Design review of the part built by this model. Coordinates are the model's own, in mm. Face numbers are marked on the shaded views. A direction names the side the tool comes from. Coordinates: 2 decimals unless noted, no trailing zeros. Loops run counter-clockwise (first coordinate to the right, second up) from the corner with the lowest first, then second, coordinate; pieces in that order, holes last. Notation, with made-up numbers: (77.5, 62) -> (105.5, 62) arc R21 cw to (105.5, 67) -> close; hole circle Ø2 at (-37.5, 58). An arc over 180 degrees is marked (long way). One line per item, written item: value. Start each with the question number.
1. Machinability: for the marked faces 1, 2 and 3, which of the approach directions +Z, -Z, +X, -X, +Y, -Y give a long, thin tool a straight path to every point of the face, cutting with its end or side? Answer none if there is none.
2. Draft analysis for pull direction X (two halves, no side actions). For the marked faces 4, 5, 6 and 7, state which applies: pulls with the +X half, pulls with the -X half, needs draft (parallel to the pull), parting line crosses it, or undercut.
3. For probe 1 along Y at (x, z) = (5, -9.25); probe 2 along Y at (x, z) = (-11, -4.25); probe 3 along Z at (x, y) = (0, -6.9), list the stretches that pass through material, from the lowest coordinate up.
4. Add section A-A on z = 0. Give the number of separate pieces and of enclosed holes in the cut face, plus the area to 3 significant figures.
5. Add section B-B on x = -6. Write out the cut boundary in (y, z).
6. Insertion check: pin 1 (2 mm diameter, centred on y = -54.5, z = -9, fed in from +X); pin 2 (0.8 mm diameter, centred on x = -17, z = 0, fed in from -Y); pin 3 (1.2 mm diameter, centred on x = -11.5, y = -45, fed in from +Z). Each pin has a flat end and moves straight along its axis. Give the tip position at first contact, or say it passes through.
7. Add section C-C on y = -25. Write out the cut boundary in (x, z), plus the area to 3 significant figures.
8. Add section D-D on z = -13. Write out the cut boundary in (x, y).
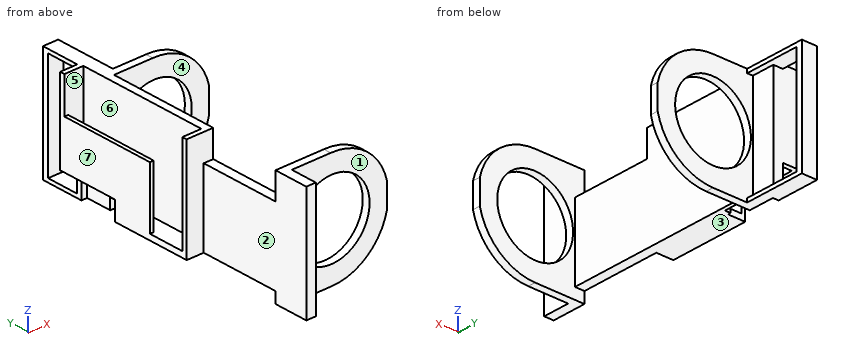
Autodesk Inventor part; units mm, degrees
ref_plane "YZ Plane" through (0, 0, 0) normal (1, 0, 0) x (0, 1, 0)
ref_plane "XZ Plane" through (0, 0, 0) normal (0, 1, 0) x (-1, 0, 0)
ref_plane "XY Plane" through (0, 0, 0) normal (0, 0, 1) x (1, 0, 0)
sketch "Sketch1" plane through (0, 0, 0) normal (0, 1, 0) x (-1, 0, 0)
  line L0 (13, 14.9495) -> (0, 14.9495)
  line L1 (0, -14.9505) -> (13, -14.9505)
  line L2 (13, -14.9505) -> (13, 14.9495)
  arc A0 (-14.7414, -2.4918) -> (0, -14.9505) centre (0, 0) ccw
  arc A1 (0.2506, 14.9495) -> (-14.7414, -2.4918) centre (-0.0002, 0.001) ccw
  point P0 (13, -0.0005)
  dimension "d0" = 29.9
  dimension "d1" = 0
  dimension "d2" = 0
extrude "Extrusion1" add sketch "Sketch1" against normal blind 60
sketch "Sketch2" plane through (0, -60, 0) normal (0, -1, 0) x (1, 0, 0)
  circle A0 centre (0, 0) radius 10
  dimension "d5" = 20
extrude "Extrusion2" cut sketch "Sketch2" against normal through all
sketch "Sketch3" plane through (0, 0, 0) normal (0, 1, 0) x (1, 0, 0)
  line L0 (-13, -14.9495) -> (-13, 14.9505)
  line L1 (-0.2506, -14.9495) -> (-13, -14.9495)
  line L2 (-13, 14.9505) -> (-10.5, 14.9505)
  line L3 (-10.5, 14.9505) -> (-10.5, -14.9495)
  line L4 (-10.5, -14.9495) -> (-13, -14.9495)
  line L5 (-13, -14.9495) -> (-13, 14.9505)
  point P0 (0, 0)
  point P1 (0, -15)
  dimension "d8" = 2.5
extrude "Extrusion3" add sketch "Sketch3" against normal blind 67
sketch "Sketch4" plane through (-10.5, -67, 14.9495) normal (1, 0, 0) x (0, 0, -1)
  line L0 (-3.796, 59) -> (37.1499, 59)
  line L1 (37.1499, 59) -> (37.1499, 9)
  line L2 (37.1499, 9) -> (-3.796, 9)
  line L3 (-3.796, 9) -> (-3.796, 59)
  line L4 (29.9, 67) -> (0, 67)
  line L5 (0, 7) -> (29.9, 7)
  point P0 (14.9495, 67)
  dimension "d31" = 2
  dimension "d44" = 50
extrude "Extrusion4" cut sketch "Sketch4" along normal through all
sketch "Sketch5" plane through (0, 0, 0) normal (0, 1, 0) x (1, 0, 0)
  line L0 (-13, 14.9505) -> (-13, -14.9495)
  line L1 (-10.5, 14.9505) -> (0, 14.9505)
  line L2 (-13, -14.9495) -> (-9, -14.9495)
  line L3 (-9, -14.9495) -> (-9, 14.9505)
  line L4 (-9, 14.9505) -> (-13, 14.9505)
  line L5 (-13, 14.9505) -> (-13, -14.9495)
  point P0 (0, 0)
  dimension "d13" = 4
extrude "Extrusion5" add sketch "Sketch5" along normal blind 10
sketch "Sketch6" plane through (-9, 0, 4.3589) normal (1, 0, 0) x (0, 0, -1)
  line L0 (0, 0) -> (-10.5906, 0)
  line L1 (-9.5906, 0) -> (18.3094, 0)
  line L2 (18.3094, 0) -> (18.3094, 8.5)
  line L3 (18.3094, 8.5) -> (-9.5906, 8.5)
  line L4 (-9.5906, 8.5) -> (-9.5906, 0)
  line L5 (19.3094, 0) -> (19.3094, 10)
  line L6 (-10.5906, 0) -> (-10.5906, 10)
  line L7 (-10.5906, 10) -> (19.3094, 10)
  point P0 (4.3589, 0)
  point P1 (19.3094, 5)
  dimension "d35" = 1
  dimension "d36" = 1
  dimension "d37" = 1.5
extrude "Extrusion6" cut sketch "Sketch6" against normal through all
sketch "Sketch7" plane through (-13, -67, -14.9505) normal (-1, 0, 0) x (0, 0, 1)
  line L0 (29.9, 67) -> (2.9, 67)
  line L1 (2.9, 67) -> (2.9, 30)
  line L2 (2.9, 30) -> (29.9, 30)
  line L3 (29.9, 30) -> (29.9, 67)
  line L4 (28.9, 67) -> (1, 67)
  line L5 (29.9, 0) -> (29.9, 77)
  line L6 (0, 0) -> (0, 77)
  point P0 (14.9505, 67)
  dimension "d54" = 37
  dimension "d55" = 27
  dimension "d57" = 0
  dimension "d60" = 0
extrude "Extrusion7" add sketch "Sketch7" along normal blind 4.5
sketch "Sketch8" plane through (-17.5, -67, -14.9505) normal (-1, 0, 0) x (0, 0, 1)
  line L0 (4.4, 65.75) -> (29.9, 65.75)
  line L1 (29.9, 65.75) -> (29.9, 31.25)
  line L2 (29.9, 31.25) -> (4.4, 31.25)
  line L3 (4.4, 31.25) -> (4.4, 65.75)
  line L4 (29.9, 30) -> (29.9, 67)
  line L5 (2.9, 30) -> (29.9, 30)
  point P0 (14.9505, 67)
  dimension "d61" = 0
  dimension "d62" = 34.5
  dimension "d63" = 25.5
  dimension "d64" = 1.25
extrude "Extrusion8" cut sketch "Sketch8" against normal blind 5
sketch "Sketch10" plane through (-10.5, -67, 14.9495) normal (1, 0, 0) x (0, 0, -1)
  line L0 (1, 67) -> (28.9, 67)
  line L1 (28.9, 67) -> (28.9, 61)
  line L2 (28.9, 61) -> (1, 61)
  line L3 (1, 61) -> (1, 67)
  line L4 (30, 59) -> (0, 59)
  line L5 (29.9, 67) -> (29.9, 77)
  line L6 (0, 67) -> (0, 77)
  point P0 (14.9495, 67)
  point P1 (1, 64)
  dimension "d45" = 2
  dimension "d46" = 6
  dimension "d48" = 1
  dimension "d50" = 1
extrude "Extrusion10" cut sketch "Sketch10" along normal through all
sketch "Sketch11" plane through (-9, 0, -14.9505) normal (1, 0, 0) x (0, 0, -1)
  line L0 (0, -67) -> (0, 10)
  line L1 (-30, 0) -> (-30, -8)
  line L2 (0, 1.2785) -> (-30, 1.2785)
  line L3 (-30, 1.2785) -> (-30, -6)
  line L4 (-30, -6) -> (0, -6)
  line L5 (0, -6) -> (0, 1.2785)
  line L6 (0, -8) -> (-30, -8)
  point P0 (-14.9505, 0)
  point P1 (0, -6)
  dimension "d51" = 2
extrude "Extrusion11" cut sketch "Sketch11" along normal through all contours L4 L1 L3 L2 L0
sketch "Sketch12" plane through (-17.5, -67, -14.9505) normal (-1, 0, 0) x (0, 0, 1)
  line L0 (2.9, 30) -> (2.9, 67)
  line L1 (2.9, 67) -> (20.4, 67)
  line L2 (20.4, 67) -> (20.4, 40.75)
  line L3 (20.4, 40.75) -> (2.9, 40.75)
  line L4 (2.9, 40.75) -> (2.9, 67)
  line L5 (4.4, 31.25) -> (4.4, 65.75)
  line L6 (4.4, 65.75) -> (29.9, 65.75)
  point P0 (14.9505, 67)
  point P1 (2.9, 40.75)
  dimension "d67" = 16
  dimension "d68" = 25
extrude "Extrusion12" add sketch "Sketch12" against normal blind 1
sketch "Sketch13" plane through (-13, -35.75, 14.9495) normal (-1, 0, 0) x (0, 0, 1)
  line L0 (0, 0) -> (-25.5, 0)
  line L1 (0, 0) -> (-7, 0)
  line L2 (-7, 0) -> (-7, 13)
  line L3 (-7, 13) -> (0, 13)
  line L4 (0, 13) -> (0, 0)
  point P0 (-14.9495, 35.75)
  dimension "d76" = 7
  dimension "d77" = 13
extrude "Extrusion13" [suppressed]
sketch "Sketch14" plane through (-17.5, -67, -14.9505) normal (-1, 0, 0) x (0, 0, 1)
  line L0 (7.9, 67) -> (2.9, 67)
  line L1 (2.9, 67) -> (2.9, 51)
  line L2 (2.9, 51) -> (7.9, 51)
  line L3 (7.9, 51) -> (7.9, 67)
  line L4 (2.9, 67) -> (2.9, 30)
  line L5 (29.9, 67) -> (2.9, 67)
  point P0 (14.9505, 67)
  dimension "d73" = 16
  dimension "d74" = 0
  dimension "d75" = 5
  dimension "d113" = 0
extrude "Extrusion14" cut sketch "Sketch14" against normal up to surface (4.5 mm away)
sketch "Sketch15" plane through (-13, -67, -14.9505) normal (-1, 0, 0) x (0, 0, 1)
  line L0 (29.9, 9) -> (0, 9)
  line L1 (0, 59) -> (2.9, 59)
  line L2 (2.9, 59) -> (2.9, 9)
  line L3 (2.9, 9) -> (0, 9)
  line L4 (0, 9) -> (0, 59)
  line L5 (2.9, 51) -> (2.9, 30)
  line L6 (0, 0) -> (0, 77)
  point P0 (14.9505, 67)
  dimension "d90" = 0
  dimension "d91" = 0
extrude "Extrusion15" cut sketch "Sketch15" against normal through all
sketch "Sketch16" plane through (-13, -67, -14.9505) normal (-1, 0, 0) x (0, 0, 1)
  line L0 (29.9, 30) -> (2.9, 30)
  line L1 (29.9, 9) -> (22.9, 9)
  line L2 (22.9, 9) -> (22.9, 30)
  line L3 (22.9, 30) -> (29.9, 30)
  line L4 (29.9, 30) -> (29.9, 9)
  line L5 (29.9, 0) -> (29.9, 30)
  point P0 (14.9505, 67)
  dimension "d82" = 0
  dimension "d83" = 7
extrude "Extrusion16" cut sketch "Sketch16" against normal through all
sketch "Sketch18" plane through (-10.5, -6, 13.9495) normal (0, 1, 0) x (1, 0, 0)
  line L0 (26.137, 9.211) -> (25.1, 9.211)
  line L1 (25.1, 9.211) -> (25.1, 19.211)
  line L2 (25.1, 19.211) -> (26.137, 19.211)
  line L3 (26.137, 19.211) -> (26.137, 9.211)
  arc A0 (10.5, -1) -> (10.5, 29) centre (10.5, 14) ccw
  point P0 (10.5, 13.9495)
  point P1 (25.1, 14.211)
  point P2 (25.5, 14)
  point P3 (25.6185, 19.211)
  point P4 (25.6185, 9.211)
  dimension "d88" = 10
  dimension "d89" = 14.6
extrude "Extrusion17" cut sketch "Sketch18" against normal through all
sketch "Sketch19" plane through (-13, -8, -14.9505) normal (-1, 0, 0) x (0, 0, 1)
  line L0 (20.4, 6.75) -> (29.9, 6.75)
  line L1 (-1.6421, -7.2479) -> (7.9, -7.2479)
  line L2 (7.9, -7.2479) -> (7.9, 6.75)
  line L3 (7.9, 6.75) -> (-1.6421, 6.75)
  line L4 (-1.6421, 6.75) -> (-1.6421, -7.2479)
  point P0 (14.9505, 8)
  point P1 (2.9, 6.75)
  point P2 (2.9, 6.75)
extrude "Extrusion18" cut sketch "Sketch19" against normal blind 1.5
properties part number "Part4-2option"
Worked answers:
1. face 1: +Z, -Z, +X, -Y
1. face 2: +Z, -Z, -X, -Y
1. face 3: -Z, +X, -X
2. face 4: needs draft
2. face 5: undercut
2. face 6: undercut
2. face 7: pulls with the -X half
3. probe 1: y = -60 to -58, -8 to -6
3. probe 2: y = -67 to 0, 8.5 to 10
3. probe 3: z = -14.95 to -10, 10 to 14.95
4. separate pieces: 4
4. enclosed holes: 0
4. area: 213 mm²
5. outline: (-60, -14.95) -> (-58, -14.95) -> (-58, -8) -> (-60, -8) -> close; (-60, 8) -> (-58, 8) -> (-58, 14.95) -> (-60, 14.95) -> close; (-8, -14.95) -> (-6, -14.95) -> (-6, -8) -> (-8, -8) -> close; (-8, 8) -> (-6, 8) -> (-6, 14.95) -> (-8, 14.95) -> close
6. pin 1: stops at x = -10.5
6. pin 2: stops at y = -37
6. pin 3: stops at z = 7.95
7. outline: (-17.5, -12.05) -> (-10.5, -12.05) -> (-10.5, 14.95) -> (-12.5, 14.95) -> (-12.5, -10.55) -> (-16.5, -10.55) -> (-16.5, 5.45) -> (-17.5, 5.45) -> close
7. area: 77.5 mm²
8. outline: (-13, -67) -> (-10.5, -67) -> (-10.5, -60) -> (7.38, -60) -> (7.38, -58) -> (-13, -58) -> close; (-13, -1.25) -> (-11.5, -1.25) -> (-11.5, -8) -> (7.38, -8) -> (7.38, -6) -> (-10.5, -6) -> (-10.5, 0) -> (-13, 0) -> close; (-13, 8.5) -> (-9, 8.5) -> (-9, 10) -> (-13, 10) -> close
